Part model, mm, in its own coordinate system. A direction names the side the tool comes from. Give positions to 0.01 mm unless a question says otherwise; leave off trailing zeros. Order: outer loops, then holes, each group sorted by start corner. A loop starts at its lowest first (then second) coordinate and runs counter-clockwise, first axis right, second up. Notation, with made-up numbers: (4, 45.5) - (39, 45.5) arc R24 ccw to (39, 77.5) - close; hole circle Ø4 at (-15, 62.25). An arc over 180 degrees is marked (long way). One line per item, written item: value.
```python
from build123d import *

# Parameters (mm, degrees)
SKETCH1_W               = 266.7
SKETCH1_H               = 241.3
BOSS_EXTRUDE1_DEPTH     = 25.4
SKETCH2_W               = 25.4
SKETCH2_H               = 241.3
BOSS_EXTRUDE2_DEPTH     = 215.9
FILLET1_R               = 12.7
CUT_EXTRUDE1_DEPTH      = 420.484671949
CUT_EXTRUDE1_DEPTH_BACK = 420.484671949
SKETCH4_R               = 16.6751
CUT_EXTRUDE2_DEPTH      = 418.943859924
CUT_EXTRUDE2_DEPTH_BACK = 418.943859924
SKETCH5_R               = 16.6751


with BuildPart() as part:
    # Sketch1 → Boss-Extrude1 (new body)
    with BuildSketch(Plane(origin=(0, 0, 0), x_dir=(1, 0, 0), z_dir=(0, 1, 0))):
        with Locations((133.35, -120.65)):
            Rectangle(SKETCH1_W, SKETCH1_H)
    extrude(amount=BOSS_EXTRUDE1_DEPTH)

    # Sketch2 → Boss-Extrude2 (add)
    with BuildSketch(Plane(origin=(0, 25.4, 0), x_dir=(1, 0, 0), z_dir=(0, 1, 0))):
        with Locations((254, -120.65)):
            Rectangle(SKETCH2_W, SKETCH2_H)
    extrude(amount=BOSS_EXTRUDE2_DEPTH)

    # Fillet1
    fillet1_edges = [part.edges().sort_by_distance(p)[0] for p in [
        (241.3, 25.4, 120.65),
        (266.7, 0, 120.65),
    ]]
    fillet(fillet1_edges, radius=FILLET1_R)

    # Sketch4 → Cut-Extrude1 (cut, two sides: drawn at the far end of the back side and taken through both)
    with BuildSketch(Plane(origin=(0, 25.4, 0), x_dir=(1, 0, 0), z_dir=(0, 1, 0)).offset(-CUT_EXTRUDE1_DEPTH_BACK)):
        with Locations(Location((25.4, -215.9, 0), (0, 0, 270))):
            Circle(SKETCH4_R)
        with Locations(Location((215.9, -215.9, 0), (0, 0, 270))):
            Circle(SKETCH4_R)
        with Locations(Location((25.4, -25.4, 0), (0, 0, 270))):
            Circle(SKETCH4_R)
        with Locations(Location((215.9, -25.4, 0), (0, 0, 270))):
            Circle(SKETCH4_R)
    extrude(amount=CUT_EXTRUDE1_DEPTH + CUT_EXTRUDE1_DEPTH_BACK, mode=Mode.SUBTRACT)

    # Sketch5 → Cut-Extrude2 (cut, two sides: drawn at the far end of the back side and taken through both)
    with BuildSketch(Plane.ZY.offset(-241.3).offset(-CUT_EXTRUDE2_DEPTH_BACK)):
        with Locations((25.4, 63.5)):
            Circle(SKETCH5_R)
        with Locations((25.4, 203.2)):
            Circle(SKETCH5_R)
        with Locations((215.9, 63.5)):
            Circle(SKETCH5_R)
        with Locations((215.9, 203.2)):
            Circle(SKETCH5_R)
    extrude(amount=CUT_EXTRUDE2_DEPTH + CUT_EXTRUDE2_DEPTH_BACK, mode=Mode.SUBTRACT)


solid = part.part
```
1) Which spindle directions (+Z, -Z, +X, -X, +Y, -Y) get a long thin tool onto all of the face, cutting with end or side? Do faces 4 (the face through (19, 12.5, 231.3)), 5 (the face through (241.3, 138, 122)). Say none if no direction does.
Answer:
face 4: +Y, -Y
face 5: +Z, -Z, -X, +Y
2) Drop flat-ended pins along their axis: P1, Ø1.5, axis at y = 93, z = 84.5, coming from the -X side; P2, Ø4, axis at x = 147.5, z = 216, coming from the +Y side; P3, Ø20, axis at x = 25.4, z = 215.9, coming from the -Y side. Give the stop position or say it passes through.
Answer:
P1: stops at x = 241.3
P2: stops at y = 25.4
P3: passes through
3) Slice it at D-D on x = 247.5. Write the cut outline in (y, z), then the cut area to 3 significant figures.
Answer:
outline: (0, 0) - (241.3, 0) - (241.3, 241.3) - (0, 241.3) - close; hole circle Ø33.35 at (63.5, 25.4); hole circle Ø33.35 at (63.5, 215.9); hole circle Ø33.35 at (203.2, 25.4); hole circle Ø33.35 at (203.2, 215.9)
area: 54,700 mm2
4) Slice it at C-C on z = 25.4. Write the cut outline in (x, y), then the cut area to 3 significant figures.
Answer:
outline: (0, 0) - (8.72, 0) - (8.72, 25.4) - (0, 25.4) - close; (42.08, 0) - (199.22, 0) - (199.22, 25.4) - (42.08, 25.4) - close; (232.58, 0) - (254, 0) arc R12.7 ccw to (266.7, 12.7) - (266.7, 46.82) - (241.3, 46.82) - (241.3, 38.1) arc R12.7 cw to (232.58, 26.04) - close; (241.3, 80.18) - (266.7, 80.18) - (266.7, 186.52) - (241.3, 186.52) - close; (241.3, 219.88) - (266.7, 219.88) - (266.7, 241.3) - (241.3, 241.3) - close
area: 8,870 mm2
5) Wall check: line 1 along Z through (x, y) = (25, 17); line 2 along X through (y, z) = (15, 215.9); line 3 along Z through (x, y) = (215, 8). Give the ranges that are in metal, low to high. Write a range as [from, to].
Answer:
line 1: z = [0, 8.73], [42.07, 199.23], [232.57, 241.3]
line 2: x = [0, 8.72], [42.08, 199.22], [232.58, 266.7]
line 3: z = [0, 8.75], [42.05, 199.25], [232.55, 241.3]
6) Slice it at A-A on y = 63.5. Write the cut outline in (x, z).
Answer:
outline: (241.3, 0) - (266.7, 0) - (266.7, 8.72) - (241.3, 8.72) - close; (241.3, 42.08) - (266.7, 42.08) - (266.7, 199.22) - (241.3, 199.22) - close; (241.3, 232.58) - (266.7, 232.58) - (266.7, 241.3) - (241.3, 241.3) - close
7) Slice it at B-B on x = 215.9. Write the cut outline in (y, z).
Answer:
outline: (0, 0) - (25.4, 0) - (25.4, 8.72) - (0, 8.72) - close; (0, 42.08) - (25.4, 42.08) - (25.4, 199.22) - (0, 199.22) - close; (0, 232.58) - (25.4, 232.58) - (25.4, 241.3) - (0, 241.3) - close
8) Two-plate mould, pull along Y, no slides. Class faces 1 (the face through (254.178, 217.261, 224.864)), 2 (the face through (182, 22, 241.3)), 3 (the face through (263.08, 3.82, 118.96)): pulls with the +Y half, pulls with the -Y half, needs draft (parallel to the pull), parting line crosses it, or undercut.
Answer:
face 1: undercut
face 2: needs draft
face 3: pulls with the -Y half
